Geometry: final body of the model. Coordinates: model frame, mm. Give positions to 0.01 mm unless a question says otherwise; leave off trailing zeros. Write each loop counter-clockwise with the first axis right and the second up, starting at its lowest first coordinate (ties: lowest second). Pieces come first, ordered by that corner, then holes.
Q1. Draft query along Y for faces 1 (the face through (-4.3, 0.3, -9.7)), 2 (the face through (-4, -7, -6.117)). Return one class per face: pulls with the +Y half, pulls with the -Y half, needs draft (parallel to the pull), parting line crosses it, or undercut.
Q2. Cut plane B-B on z = -9.75. Return the cut outline in (x, y), plus the area to 3 significant figures.
Q3. Cut plane C-C on x = 4. Return the cut outline in (y, z), plus the area to 3 significant figures.
Q4. Cut plane D-D on y = 6. Return the cut outline in (x, z).
Q5. Line query: L1, parallel to X at y = 3.25, z = -7.6; L2, parallel to Y at x = -5.75, z = -6.35; L3, parallel to Y at x = -4.75, z = -6.9. Output: solid intervals per line, ascending.
Q6. Cut plane A-A on y = 0. Return the cut outline in (x, z), plus the area to 3 significant figures.
Q7. Pin query (flat end, axial travel): pin 1 (5 mm diameter, centred on x = -2, y = -2.5, fed in from +Z); pin 2 (6 mm diameter, centred on x = 6.5, y = -5.5, fed in from -Z); pin 3 (1.5 mm diameter, centred on x = -0.5, z = -10, fed in from +Y). Return the tip coordinate at first contact, or that it passes through.
```python
from build123d import *

# Parameters (mm, degrees)
F2_W     = 28.774573
F2_H     = 22.486091
F3_DEPTH = 12.7
F4_T     = -1
F5_R     = 0.510478
F6_DEPTH = 25.4


with BuildPart() as f1:
    # F0 (on Front) → F1 (revolve)
    with BuildSketch(Plane.XZ):
        with BuildLine():
            Line((0, 0), (0, 11))
            ThreePointArc((0, 11), (-11, 0), (0, -11))
            Line((0, -11), (0, 0))
        make_face()
    revolve(axis=Axis((0, 0, 0), (0, 0, -1)))

    # F2 (on Front) → F3 (cut, symmetric)
    with BuildSketch(Plane.XZ):
        with Locations((-1.024286, 5.125662)):
            Rectangle(F2_W, F2_H)
    extrude(amount=F3_DEPTH, both=True, mode=Mode.SUBTRACT)

    # F4
    f4_openings = [f1.faces().sort_by_distance(p)[0] for p in [
        (0, 0, -6.117383),
    ]]
    offset(amount=F4_T, openings=f4_openings)

    # F5 (on Top) → F6 (cut)
    with BuildSketch(Plane.XY):
        with Locations((-3.888461, 0)):
            Circle(F5_R)
    extrude(amount=-F6_DEPTH, mode=Mode.SUBTRACT)


solid = f1.part
```
Data:
1. face 1: undercut
1. face 2: needs draft
2. outline: circle Ø10.19 at (0, 0); hole circle Ø1.02 at (-3.89, 0); hole circle Ø4.44 at (0, 0)
2. area: 65.2 mm2
3. outline: (-8.22, -6.12) arc R10.25 ccw to (8.22, -6.12) - (6.82, -6.12) arc R9.17 cw to (-6.82, -6.12) - close
3. area: 18.7 mm2
4. outline: (-6.9, -6.12) arc R9.22 ccw to (6.9, -6.12) - (5.16, -6.12) arc R8 cw to (-5.16, -6.12) - close
5. L1: x = -7.26 to -5.63, 5.63 to 7.26
5. L2: y = -6.9 to -5.16, 5.16 to 6.9
5. L3: y = -7.13 to -5.46, 5.46 to 7.13
6. outline: (-9.14, -6.12) arc R11 ccw to (-4.4, -10.08) - (-4.4, -8.98) arc R10 cw to (-7.91, -6.12) - close; (-3.38, -10.47) arc R11 ccw to (9.14, -6.12) - (7.91, -6.12) arc R10 cw to (-3.38, -9.41) - close
6. area: 18.8 mm2
7. pin 1: stops at z = -8.22
7. pin 2: stops at z = -9.52
7. pin 3: stops at y = 5.93
